Design review of the part shown in the three views and the two pictorial views. Dimensions are in mm from the part's minimum x, y and z. A direction names the side the tool comes from. Coordinates: 2 decimals unless noted, no trailing zeros. Loops run counter-clockwise (first coordinate to the right, second up) from the corner with the lowest first, then second, coordinate; pieces in that order, holes last. Notation, with made-up numbers: (83, -30.75) -> (88, -30.75) arc R23 ccw to (88, -2.75) -> close; hole circle Ø1 at (88.25, 0). An arc over 180 degrees is marked (long way). Answer in a Markdown table with one row per item.
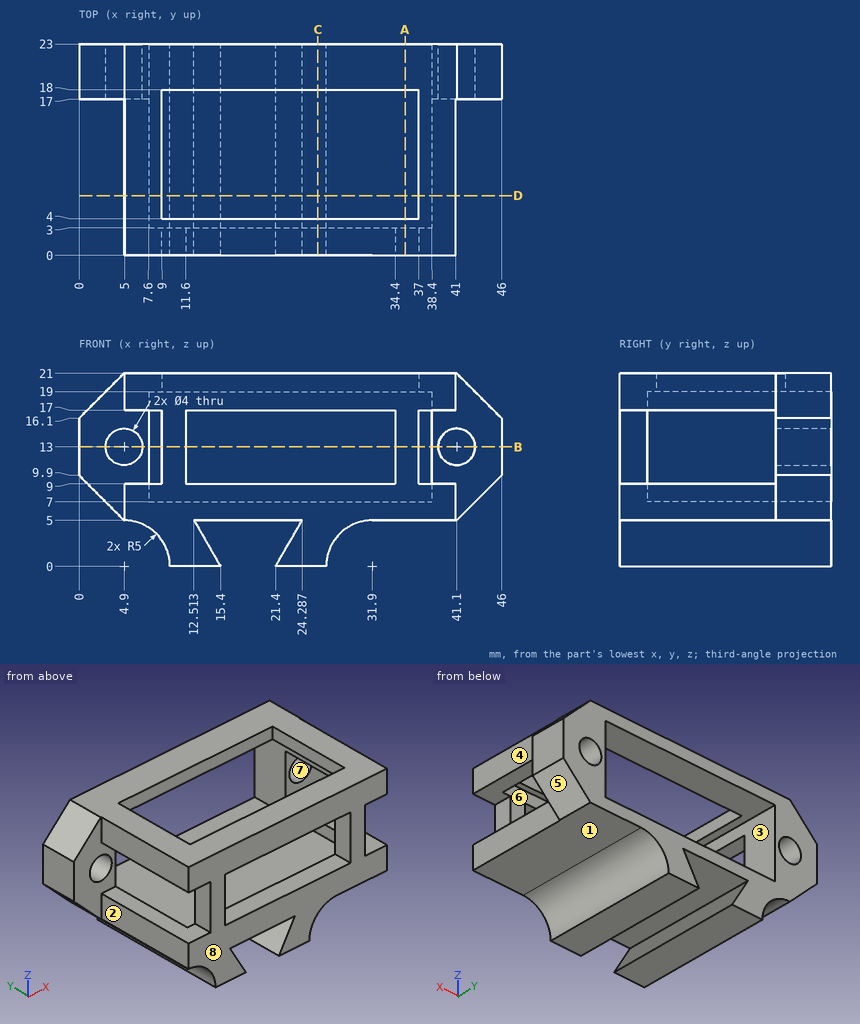
Item 1: Take a section at B-B, the plane z = 13. State the section outline as (x, y) points, and give its area (3 significant figures).
Worked answers:
| item | result |
|---|---|
| outline | (0, 17) -> (2.9, 17) -> (2.9, 23) -> (0, 23) -> close; (6.9, 17) -> (7.6, 17) -> (7.6, 23) -> (6.9, 23) -> close; (9, 0) -> (11.6, 0) -> (11.6, 3) -> (9, 3) -> close; (34.4, 0) -> (37, 0) -> (37, 3) -> (34.4, 3) -> close; (38.4, 17) -> (39.1, 17) -> (39.1, 23) -> (38.4, 23) -> close; (43.1, 17) -> (46, 17) -> (46, 23) -> (43.1, 23) -> close |
| area | 58.8 mm² |
Item 2: Insertion check: pin 1 (0.9 mm diameter, centred on y = 2, z = 14, fed in from -X); pin 2 (12 mm diameter, centred on x = 33, z = 6, fed in from -Y); pin 3 (1.2 mm diameter, centred on x = 39, y = 12.5, fed in from -Z); pin 4 (1.6 mm diameter, centred on y = 12.5, z = 19.5, fed in from -X). Each pin has a flat end and moves straight along its axis. Give the tip position at first contact, or say it passes through.
Worked answers:
| item | result |
|---|---|
| pin 1 | x = 9 |
| pin 2 | y = 0 |
| pin 3 | z = 5 |
| pin 4 | x = 5 |
Item 3: For L1, parallel to X at y = 20.65, z = 13; L2, parallel to Z at x = 4.9, y = 18.2; L3, parallel to X at y = 8.5, z = 5.25, list the stretches that pass through material, from the lowest coordinate up.
Worked answers:
| item | result |
|---|---|
| L1 | 0 to 2.9, 6.9 to 7.6, 38.4 to 39.1, 43.1 to 46 |
| L2 | 5 to 11, 15 to 21 |
| L3 | 5 to 41 |
Item 4: The part is to be moulded in two halves that separate along X. For the marked faces 5, 6, 7 and 8, say which applies: +X half, -X half, draft (parallel to the pull), parting line (faces both ways), or undercut.
Worked answers:
| item | result |
|---|---|
| face 5 | +X half |
| face 6 | undercut |
| face 7 | undercut |
| face 8 | draft |
Item 5: Take a section at D-D, the plane y = 6.5. State the section outline as (x, z) points.
Worked answers:
| item | result |
|---|---|
| outline | (4.9, 5) arc R5 cw to (9.9, 0) -> (15.4, 0) -> (12.51, 5) -> (24.29, 5) -> (21.4, 0) -> (26.9, 0) arc R5 cw to (31.9, 5) -> (41, 5) -> (41, 9) -> (38.4, 9) -> (38.4, 7) -> (7.6, 7) -> (7.6, 9) -> (5, 9) -> (5, 5) -> close; (5, 17) -> (7.6, 17) -> (7.6, 19) -> (9, 19) -> (9, 21) -> (5, 21) -> close; (37, 19) -> (38.4, 19) -> (38.4, 17) -> (41, 17) -> (41, 21) -> (37, 21) -> close |
Item 6: For the marked faces 1, 2, 3 and 4, list the 3-axis set-ups (+Z, -Z, +X, -X, +Y, -Y) from which the entire face can be reached by the end or side of a thin tool; tool diameter is ignored.
Worked answers:
| item | result |
|---|---|
| face 1 | -Z, +X, +Y, -Y |
| face 2 | +Z, -X, -Y |
| face 3 | +Y |
| face 4 | +Z, -Z, +X, -Y |
Item 7: Take a section at A-A, the plane x = 35.5. State the section outline as (y, z) points.
Worked answers:
| item | result |
|---|---|
| outline | (0, 5) -> (23, 5) -> (23, 7) -> (3, 7) -> (3, 19) -> (4, 19) -> (4, 21) -> (0, 21) -> close; (18, 19) -> (23, 19) -> (23, 21) -> (18, 21) -> close |
Item 8: Take a section at C-C, the plane x = 26. State the section outline as (y, z) points.
Worked answers:
| item | result |
|---|---|
| outline | (0, 0) -> (23, 0) -> (23, 7) -> (3, 7) -> (3, 9) -> (0, 9) -> close; (0, 17) -> (3, 17) -> (3, 19) -> (4, 19) -> (4, 21) -> (0, 21) -> close; (18, 19) -> (23, 19) -> (23, 21) -> (18, 21) -> close |
